Study the drawing (mm; zero at the part's minimum x, y, z) and answer. A direction names the side the tool comes from. Coordinates: 2 decimals unless noted, no trailing zeros. Loops run counter-clockwise (first coordinate to the right, second up) from the corner with the lowest first, then second, coordinate; pieces in that order, holes last. Notation, with made-up numbers: (-20.5, 14.5) - (8.5, 14.5) arc R23 cw to (8.5, 39.5) - close; hole circle Ø5 at (49, 18). An arc over 180 degrees is marked (long way). Write each question's results on one line, items separated by ' | '. Start each with the question number.
(1) Consider line 1 (Y direction, x = 0.85, z = 5.5); line 2 (X direction, y = 15, z = 10); line 3 (Y direction, x = 17.25, z = 3). Determine where each line is inside the solid, lowest interval first. Write a range as from..to.
(2) Find section D-D on y = 5.75. Determine the outline of the cut face in (x, z).
(3) For the marked faces 4 and 5, determine the directions among +Z, -Z, +X, -X, +Y, -Y from which every point of the face is accessible in a straight line to the end or side of a thin tool.
(4) Determine the mould class of the marked faces 1, 2 and 3 for opening direction X: released by +X, released by -X, zero draft, split by the parting line, or undercut.
(5) Given pin 1 Ø3.5 at (y, z) = (5, 5.5) entering from -X; pin 2 Ø1.8 at (y, z) = (5, 5.5) entering from -X; pin 3 Ø6 at (x, z) = (10.5, 7.5) entering from +Y, each flat-ended and moving along its own axis, determine where each tip first touches the part or whether it passes through.
(6) Find section C-C on z = 10.5. Determine the outline of the cut face in (x, y).
(7) Find section B-B on z = 5.5. Determine the outline of the cut face in (x, y).
(8) Find section A-A on y = 15. Determine the outline of the cut face in (x, z).
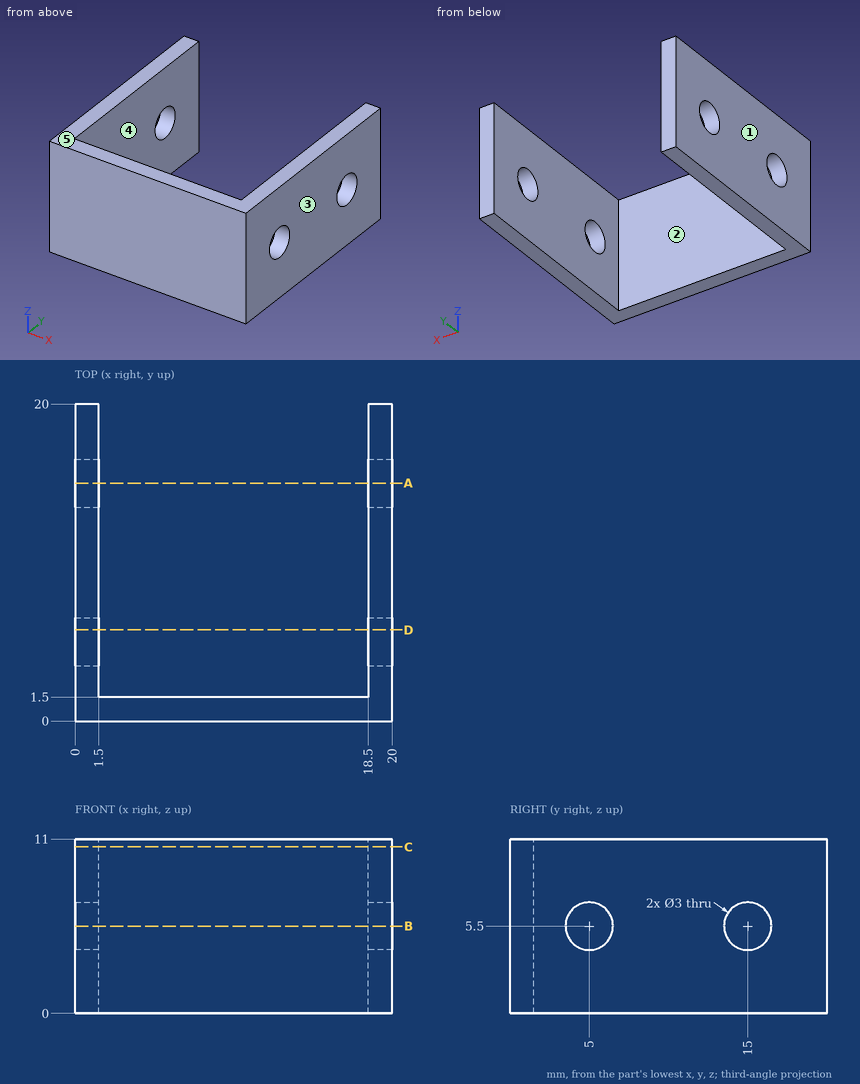
Values:
1) line 1: y = 0..3.5, 6.5..13.5, 16.5..20 | line 2: x = 0..1.5, 18.5..20 | line 3: y = 0..1.5
2) outline: (0, 0) - (1.5, 0) - (1.5, 4.2) - (0, 4.2) - close; (0, 6.8) - (1.5, 6.8) - (1.5, 11) - (0, 11) - close; (18.5, 0) - (20, 0) - (20, 4.2) - (18.5, 4.2) - close; (18.5, 6.8) - (20, 6.8) - (20, 11) - (18.5, 11) - close
3) face 4: +Z, -Z, +Y | face 5: +Z, +X, -X, +Y, -Y
4) face 1: released by -X | face 2: undercut | face 3: released by +X
5) pin 1: stops at x = 0 | pin 2: passes through | pin 3: stops at y = 1.5
6) outline: (0, 0) - (20, 0) - (20, 20) - (18.5, 20) - (18.5, 1.5) - (1.5, 1.5) - (1.5, 20) - (0, 20) - close
7) outline: (0, 0) - (20, 0) - (20, 3.5) - (18.5, 3.5) - (18.5, 1.5) - (1.5, 1.5) - (1.5, 3.5) - (0, 3.5) - close; (0, 6.5) - (1.5, 6.5) - (1.5, 13.5) - (0, 13.5) - close; (0, 16.5) - (1.5, 16.5) - (1.5, 20) - (0, 20) - close; (18.5, 6.5) - (20, 6.5) - (20, 13.5) - (18.5, 13.5) - close; (18.5, 16.5) - (20, 16.5) - (20, 20) - (18.5, 20) - close
8) outline: (0, 0) - (1.5, 0) - (1.5, 4) - (0, 4) - close; (0, 7) - (1.5, 7) - (1.5, 11) - (0, 11) - close; (18.5, 0) - (20, 0) - (20, 4) - (18.5, 4) - close; (18.5, 7) - (20, 7) - (20, 11) - (18.5, 11) - close
